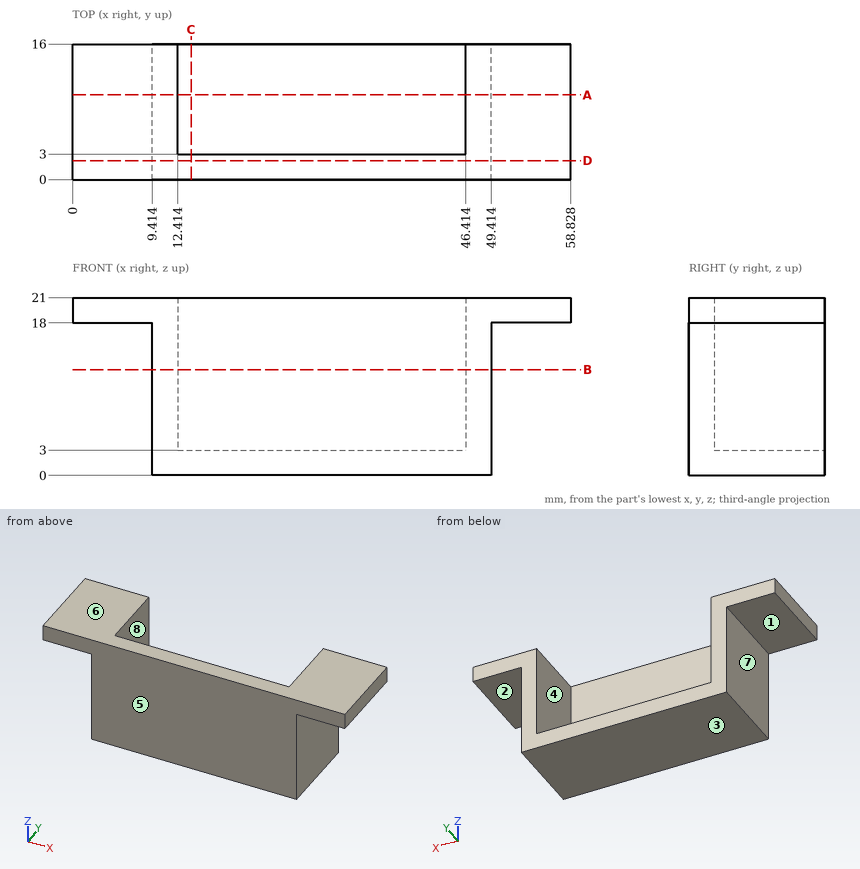
Here's the drawing with two shaded views (mm, measured from the low corner). I have some questions. A direction names the side the tool comes from. Coordinates: 2 decimals unless noted, no trailing zeros. Order: outer loops, then holes, each group sorted by start corner. A loop starts at its lowest first (then second) coordinate and runs counter-clockwise, first axis right, second up.
Item 1: For P1, Ø1, axis at y = 7, z = 16.5, coming from the -X side; P2, Ø2, axis at y = 12, z = 7, coming from the +X side; P3, Ø6.5, axis at x = 33.5, y = 12.5, coming from the +Z side, each with a flat end and sliding along its axis, tell me the tip position at first contact or that it passes through.
Result sheet:
P1: stops at x = 9.41
P2: stops at x = 49.41
P3: stops at z = 3
Item 2: I need wall thicknesses on line 1 (X direction, y = 8, z = 8.75); line 2 (X direction, y = 4.25, z = 18.5); line 3 (X direction, y = 13.25, z = 1). Which ranges of each line are inside material? Lowest first, please.
Result sheet:
line 1: x = 9.41 to 12.41, 46.41 to 49.41
line 2: x = 0 to 12.41, 46.41 to 58.83
line 3: x = 9.41 to 49.41
Item 3: If we section it at A-A on y = 10: List the corners of the cut face in (x, z) for me.
Result sheet:
outline: (0, 18) - (9.41, 18) - (9.41, 0) - (49.41, 0) - (49.41, 18) - (58.83, 18) - (58.83, 21) - (46.41, 21) - (46.41, 3) - (12.41, 3) - (12.41, 21) - (0, 21) - close
Item 4: For the marked faces 1, 2, 3, 4 and 5, which set-ups out of +Z, -Z, +X, -X, +Y, -Y let a thin tool reach every point of the face, with its end or its side?
Result sheet:
face 1: -Z, -X, +Y, -Y
face 2: -Z, +X, +Y, -Y
face 3: -Z, +X, -X, +Y, -Y
face 4: +Z, +Y
face 5: +Z, -Z, +X, -X, -Y
Item 5: If we section it at D-D on y = 2.25: List the corners of the cut face in (x, z) for me.
Result sheet:
outline: (0, 18) - (9.41, 18) - (9.41, 0) - (49.41, 0) - (49.41, 18) - (58.83, 18) - (58.83, 21) - (0, 21) - close
Item 6: If we mould it in two halves opening along X, with no side actions, what happens to the marked faces 6, 7 and 8? For each: +X half, -X half, draft (parallel to the pull), parting line (faces both ways), or undercut.
Result sheet:
face 6: draft
face 7: -X half
face 8: undercut
Item 7: If we section it at B-B on z = 12.5: List the corners of the cut face in (x, y) for me, plus the area to 3 significant figures.
Result sheet:
outline: (9.41, 0) - (49.41, 0) - (49.41, 16) - (46.41, 16) - (46.41, 3) - (12.41, 3) - (12.41, 16) - (9.41, 16) - close
area: 198 mm2
Item 8: If we section it at C-C on x = 14: List the corners of the cut face in (y, z) for me.
Result sheet:
outline: (0, 0) - (16, 0) - (16, 3) - (3, 3) - (3, 21) - (0, 21) - close
